Can you work these out from the model? Positions are in its coordinate system, mm. Face numbers are marked on the shaded views. A direction names the side the tool comes from. Give positions to 0.01 mm unless a question says otherwise; leave off trailing zeros. Write each loop counter-clockwise with the first axis right and the second up, starting at its lowest first coordinate (ties: lowest second). Pieces come first, ordered by that corner, then holes. Notation, with made-up numbers: (-2.75, 81) - (42.25, 81) arc R23 ccw to (42.25, 101) - close; hole circle Ø3 at (35, -3). An arc over 180 degrees is marked (long way). Use a Markdown table: item, result. Add a question column.
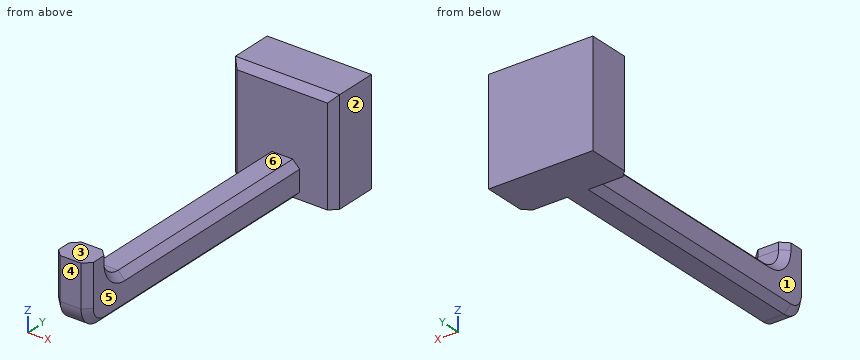
```python
from build123d import *

# Parameters (mm, degrees)
SKETCH_W        = 15
SKETCH_H        = 15
PAD_DEPTH       = 7
SKETCH001_W     = 5
SKETCH001_H     = 5
PAD001_DEPTH    = 40
SKETCH002_W     = 5
SKETCH002_H     = 4
PAD002_DEPTH    = 4
CHAMFER_SIZE    = 1
FILLET_R        = 3
CHAMFER001_SIZE = 1
CHAMFER002_SIZE = 1


with BuildPart() as part:
    # Sketch → Pad (new body)
    with BuildSketch(Plane.XZ):
        with Locations((0, -7.5)):
            Rectangle(SKETCH_W, SKETCH_H)
    extrude(amount=PAD_DEPTH)

    # Sketch001 (on Face6 of Pad) → Pad001 (join)
    with BuildSketch(Plane.XZ.offset(7)):
        with Locations((0, -12.5)):
            Rectangle(SKETCH001_W, SKETCH001_H)
    extrude(amount=PAD001_DEPTH)

    # Sketch002 (on Face7 of Pad001) → Pad002 (join)
    with BuildSketch(Plane(origin=(0, 0, -10), x_dir=(-1, 0, 0), z_dir=(0, 0, 1))):
        with Locations((0, 45)):
            Rectangle(SKETCH002_W, SKETCH002_H)
    extrude(amount=PAD002_DEPTH)

    # Chamfer
    chamfer_edges = [part.edges().sort_by_distance(p)[0] for p in [
        (0, -7, 0),
        (-7.5, -7, -7.5),
        (7.5, -7, -7.5),
    ]]
    chamfer(chamfer_edges, length=CHAMFER_SIZE)

    # Fillet
    fillet_edges = [part.edges().sort_by_distance(p)[0] for p in [
        (0, -43, -10),
        (0, -47, -15),
    ]]
    fillet(fillet_edges, radius=FILLET_R)

    # Chamfer001
    chamfer001_edges = [part.edges().sort_by_distance(p)[0] for p in [
        (2.5, -25.5, -15),
        (-2.5, -25.5, -15),
    ]]
    chamfer(chamfer001_edges, length=CHAMFER001_SIZE)

    # Chamfer002
    chamfer002_edges = [part.edges().sort_by_distance(p)[0] for p in [
        (2.5, -23.5, -10),
        (-2.5, -23.5, -10),
    ]]
    chamfer(chamfer002_edges, length=CHAMFER002_SIZE)


solid = part.part
```
Q1. Suppose I cut it at B-B (y = -25). Please give me the cut outline in (x, z), and give its area (3 significant figures).
Q2. Suppose I cut it at D-D (z = -2.5). Please give me the cut outline in (x, y), and give its area (3 significant figures).
Q3. If I drill on probe 1 along Y at (x, z) = (5.5, -1.75); probe 2 along X at (y, z) = (-34, -13.75); probe 3 along Z at (x, y) = (-0.75, -13), over which ranges is the centre line in solid material (lowest first)? Write a range as [from, to].
Q4. On a 3-axis mill with a long thin cutter (end or side, diameter ignored), from which of +Z, -Z, +X, -X, +Y, -Y can I reach the whole of each face in a straight line? I mean the marked faces 1, 2 and 3. Say none if no direction works.
Q5. If we mould it in two halves opening along Y, with no side actions, what happens to the marked faces 4, 5 and 6? For each: released by +Y, released by -Y, zero draft, split by the parting line, or undercut.
Q6. Suppose I cut it at C-C (x = -0.75). Please give me the cut outline in (y, z), and give its area (4 significant figures).
Q7. I'm going to push flat-ended pins straight in: P1, Ø2.5, axis at y = -30, z = -9.5, coming from the -X side; P2, Ø5, axis at x = 3, y = -33.5, coming from the +Z side; P3, Ø3, axis at x = -0.5, y = -44.5, coming from the +Z side. Where does each tip first touch, or does it pass through?
Q8. Suppose I cut it at A-A (z = -6.5). Please give me the cut outline in (x, y).
Derived:
| question | item | result |
|---|---|---|
| 1 | outline | (-2.5, -14) - (-1.5, -15) - (1.5, -15) - (2.5, -14) - (2.5, -11) - (1.5, -10) - (-1.5, -10) - (-2.5, -11) - close |
| 1 | area | 23.0 mm² |
| 2 | outline | (-7.5, -6) - (-6.5, -7) - (6.5, -7) - (7.5, -6) - (7.5, 0) - (-7.5, 0) - close |
| 2 | area | 104 mm² |
| 3 | probe 1 | [-7, 0] |
| 3 | probe 2 | [-2.5, 2.5] |
| 3 | probe 3 | [-15, -10] |
| 4 | face 1 | +Z, -Z, -X, -Y |
| 4 | face 2 | +Z, -Z, +X, +Y, -Y |
| 4 | face 3 | +Z, +X, -X, -Y |
| 5 | face 4 | released by -Y |
| 5 | face 5 | zero draft |
| 5 | face 6 | undercut |
| 6 | outline | (-47, -12) arc R3 ccw to (-44, -15) - (0, -15) - (0, 0) - (-6, 0) - (-7, -1) - (-7, -10) - (-40, -10) arc R3 cw to (-43, -7) - (-43, -6) - (-47, -6) - close |
| 6 | area | 320.5 mm² |
| 7 | P1 | x = -2.25 |
| 7 | P2 | z = -10 |
| 7 | P3 | z = -6 |
| 8 | outline | (-7.5, -6) - (-6.5, -7) - (6.5, -7) - (7.5, -6) - (7.5, 0) - (-7.5, 0) - close; (-2.5, -46) - (-1.5, -47) - (1.5, -47) - (2.5, -46) - (2.5, -44) - (1.5, -43) - (-1.5, -43) - (-2.5, -44) - close |
